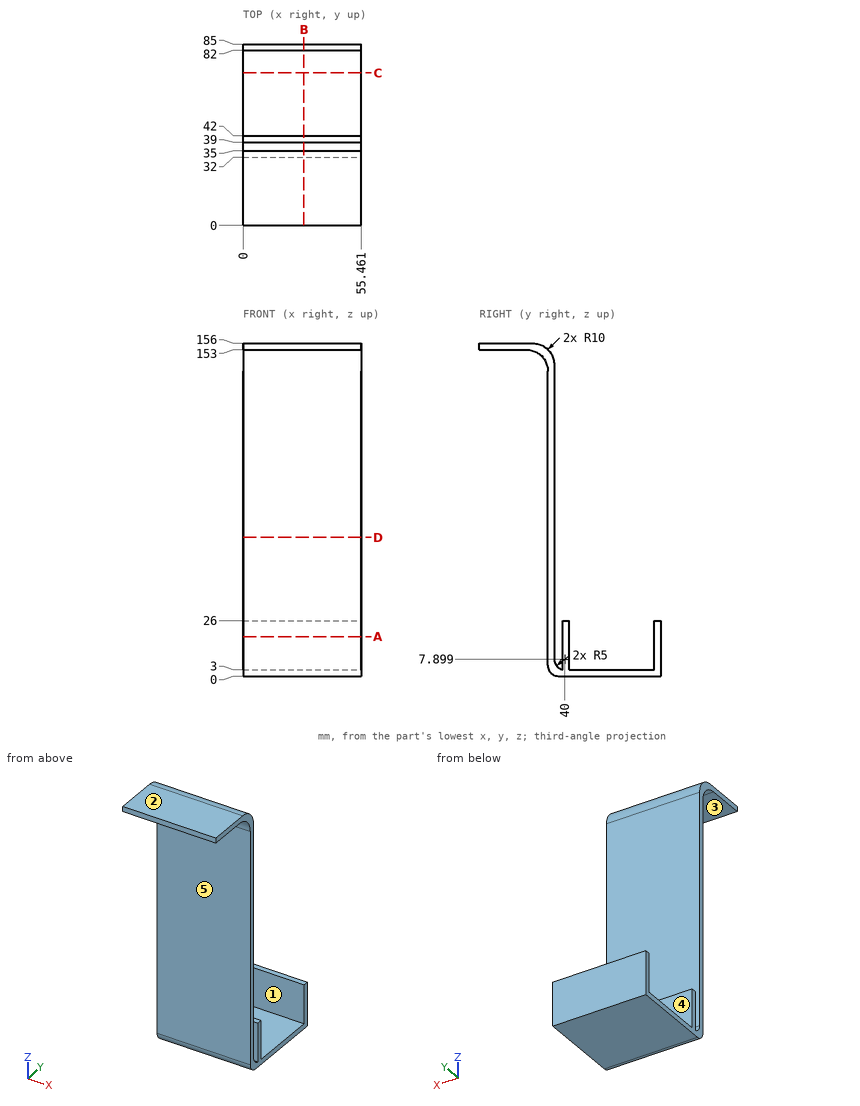
Print and shaded views of the part. All mm, measured from the part's lowest x, y and z. A direction names the side the tool comes from. Coordinates: 2 decimals unless noted, no trailing zeros. Loops run counter-clockwise (first coordinate to the right, second up) from the corner with the lowest first, then second, coordinate; pieces in that order, holes last. Notation, with made-up numbers: (-6, 69.25) -> (1, 69.25) arc R22 cw to (1, 99.25) -> close; hole circle Ø5 at (5, 23.25). An arc over 180 degrees is marked (long way). Use a Markdown table: item, result. Add a question column.
Item 1: Band-saw the part on B-B on x = 28.5. Write the cut outline in (y, z).
Item 2: Band-saw the part on A-A on z = 18.5. Write the cut outline in (x, y), plus the area to 3 significant figures.
Item 3: Which spindle directions (+Z, -Z, +X, -X, +Y, -Y) get a long thin tool onto all of the face, cutting with end or side? Do the marked faces 1 and 2. Say none if no direction does.
Item 4: Band-saw the part on D-D on z = 65. Write the cut outline in (x, y), plus the area to 3 significant figures.
Item 5: Probe probe 1 along Z at (x, y) = (12.5, 59); probe 2 along Y at (x, z) = (26.5, 132.5); probe 3 along Z at (x, y) = (51, 11). List the from-to ranges inside material, lowest first.
Item 6: Pull direction Y, two halves, no side cores. Call the marked faces 3, 4 and 5: +Y half, -Y half, draft (parallel to the pull), parting line (faces both ways), or undercut.
Item 7: Band-saw the part on C-C on y = 71.5. Write the cut outline in (x, z), plus the area to 3 significant figures.
Item 8: Flat gauge pins, fed straight in: P1, Ø24, axis at x = 29.5, y = 6.5, coming from the -Z side; P2, Ø5, axis at x = 13, y = 31, coming from the +Z side; P3, Ø18.5, axis at x = 32.5, z = 10, coming from the -Y side. Where does each tip first touch, or does it go through?
Geometry says:
| question | item | result |
|---|---|---|
| 1 | outline | (0, 153) -> (22, 153) arc R10 cw to (32, 143) -> (32, 5) arc R5 ccw to (37, 0) -> (85, 0) -> (85, 26) -> (82, 26) -> (82, 3) -> (42, 3) -> (42, 26) -> (39, 26) -> (39, 3) arc R5 cw to (35, 7.9) -> (35, 146) arc R10 ccw to (25, 156) -> (0, 156) -> close |
| 2 | outline | (0, 32) -> (55.46, 32) -> (55.46, 35) -> (0, 35) -> close; (0, 39) -> (55.46, 39) -> (55.46, 42) -> (0, 42) -> close; (0, 82) -> (55.46, 82) -> (55.46, 85) -> (0, 85) -> close |
| 2 | area | 499 mm² |
| 3 | face 1 | +Z, +X, -X |
| 3 | face 2 | +Z, +X, -X, +Y, -Y |
| 4 | outline | (0, 32) -> (55.46, 32) -> (55.46, 35) -> (0, 35) -> close |
| 4 | area | 166 mm² |
| 5 | probe 1 | 0 to 3 |
| 5 | probe 2 | 32 to 35 |
| 5 | probe 3 | 153 to 156 |
| 6 | face 3 | draft |
| 6 | face 4 | undercut |
| 6 | face 5 | -Y half |
| 7 | outline | (0, 0) -> (55.46, 0) -> (55.46, 3) -> (0, 3) -> close |
| 7 | area | 166 mm² |
| 8 | P1 | z = 153 |
| 8 | P2 | z = 155.37 |
| 8 | P3 | y = 32 |
